Geometry: final body of the model. Coordinates: model frame, mm. A direction names the side the tool comes from. Round coordinates to 2 decimals unless told otherwise and drop trailing zeros. Loops run counter-clockwise (first coordinate to the right, second up) from the corner with the lowest first, then second, coordinate; pieces in that order, holes last. Notation, with made-up numbers: M 12,52.5 L 60,52.5 A20 cw 60,83.5 Z; hole C -9.5,54.25 d5. An arc over 180 degrees is marked long. Return JSON: item names as keys, results as strings.
from build123d import *

# Parameters (mm, degrees)
CROQUIS1_W                 = 45
CROQUIS1_H                 = 45
SALIENTE_EXTRUIR1_DEPTH    = 300
CROQUIS4_W                 = 18
CROQUIS4_H                 = 34
CORTAR_EXTRUIR2_DEPTH      = 46
CROQUIS8_W                 = 35
CROQUIS8_H                 = 35
CORTAR_EXTRUIR3_DEPTH      = 301
CROQUIS9_W                 = 35
CROQUIS9_H                 = 21.174410022
CORTAR_EXTRUIR4_DEPTH      = 10
CROQUIS10_R                = 1
CORTAR_EXTRUIR5_DEPTH      = 10
CROQUIS11_W                = 45
CROQUIS11_H                = 26.387879272
CORTAR_EXTRUIR6_DEPTH      = 46
CROQUIS13_W                = 45
CROQUIS13_H                = 50
CORTAR_EXTRUIR7_DEPTH      = 23.5
CORTAR_EXTRUIR7_DEPTH_BACK = 23.5
CROQUIS14_W                = 55
CROQUIS14_H                = 55
SALIENTE_EXTRUIR2_DEPTH    = 5
CROQUIS16_R                = 1
CORTAR_EXTRUIR8_DEPTH      = 1
CORTAR_EXTRUIR8_DEPTH_BACK = 229.612120728
CROQUIS17_R                = 2.5
CROQUIS17_R_2              = 2.03
CORTAR_EXTRUIR9_DEPTH      = 6
CORTAR_EXTRUIR9_DEPTH_BACK = 51


with BuildPart() as part:
    # Croquis1 → Saliente-Extruir1 (new body)
    with BuildSketch(Plane(origin=(0, 0, 0), x_dir=(1, 0, 0), z_dir=(0, 1, 0))):
        Rectangle(CROQUIS1_W, CROQUIS1_H)
    extrude(amount=SALIENTE_EXTRUIR1_DEPTH)

    # Croquis4 → Cortar-Extruir2 (cut, through all)
    with BuildSketch(Plane.ZY.offset(22.5)):
        with Locations((13.5, 17)):
            Rectangle(CROQUIS4_W, CROQUIS4_H)
    extrude(amount=-CORTAR_EXTRUIR2_DEPTH, mode=Mode.SUBTRACT)

    # Croquis8 → Cortar-Extruir3 (cut, through all)
    with BuildSketch(Plane(origin=(0, 300, 0), x_dir=(1, 0, 0), z_dir=(0, 1, 0))):
        Rectangle(CROQUIS8_W, CROQUIS8_H)
    extrude(amount=-CORTAR_EXTRUIR3_DEPTH, mode=Mode.SUBTRACT)

    # Croquis9 → Cortar-Extruir4 (cut)
    with BuildSketch(Plane(origin=(0, 0, -22.5), x_dir=(-1, 0, 0), z_dir=(0, 0, -1))):
        with Locations((0, 260)):
            Rectangle(CROQUIS9_W, CROQUIS9_H)
    extrude(amount=-CORTAR_EXTRUIR4_DEPTH, mode=Mode.SUBTRACT)

    # Croquis10 → Cortar-Extruir5 (cut)
    with BuildSketch(Plane.XY.offset(22.5)):
        with Locations((0, 260)):
            Circle(CROQUIS10_R)
    extrude(amount=-CORTAR_EXTRUIR5_DEPTH, mode=Mode.SUBTRACT)

    # Croquis11 → Cortar-Extruir6 (cut, through all)
    with BuildSketch(Plane.XY.offset(22.5)):
        with Locations((0, 286.806060364)):
            Rectangle(CROQUIS11_W, CROQUIS11_H)
    extrude(amount=-CORTAR_EXTRUIR6_DEPTH, mode=Mode.SUBTRACT)

    # Croquis13 → Cortar-Extruir7 (cut, two sides)
    with BuildSketch(Plane(origin=(0, 0, 0), x_dir=(0, 0, -1), z_dir=(1, 0, 0))) as cortar_extruir7_sk:
        with Locations((0, 25)):
            Rectangle(CROQUIS13_W, CROQUIS13_H)
    extrude(amount=CORTAR_EXTRUIR7_DEPTH, mode=Mode.SUBTRACT)
    extrude(cortar_extruir7_sk.sketch, amount=-CORTAR_EXTRUIR7_DEPTH_BACK, mode=Mode.SUBTRACT)

    # Croquis14 → Saliente-Extruir2 (add)
    with BuildSketch(Plane.XZ.offset(-50)):
        Rectangle(CROQUIS14_W, CROQUIS14_H)
    extrude(amount=SALIENTE_EXTRUIR2_DEPTH)

    # Croquis16 → Cortar-Extruir8 (cut, two sides)
    with BuildSketch(Plane.XZ.offset(-45)) as cortar_extruir8_sk:
        with Locations((25, 25)):
            Circle(CROQUIS16_R)
        with Locations((-25, 25)):
            Circle(CROQUIS16_R)
        with Locations((-25, -25)):
            Circle(CROQUIS16_R)
        with Locations((25, -25)):
            Circle(CROQUIS16_R)
    extrude(amount=CORTAR_EXTRUIR8_DEPTH, mode=Mode.SUBTRACT)
    extrude(cortar_extruir8_sk.sketch, amount=-CORTAR_EXTRUIR8_DEPTH_BACK, mode=Mode.SUBTRACT)

    # Croquis17 → Cortar-Extruir9 (cut, two sides)
    with BuildSketch(Plane.XY.offset(22.5)) as cortar_extruir9_sk:
        with Locations((-10, 262.50260741)):
            Circle(CROQUIS17_R)
        with Locations((-10, 206.50260741)):
            Circle(CROQUIS17_R)
        with Locations((10, 262.50260741)):
            Circle(CROQUIS17_R)
        with Locations((10, 206.50260741)):
            Circle(CROQUIS17_R)
        with Locations((10, 254.10260741)):
            Circle(CROQUIS17_R_2)
        with Locations((10, 214.90260741)):
            Circle(CROQUIS17_R_2)
    extrude(amount=CORTAR_EXTRUIR9_DEPTH, mode=Mode.SUBTRACT)
    extrude(cortar_extruir9_sk.sketch, amount=-CORTAR_EXTRUIR9_DEPTH_BACK, mode=Mode.SUBTRACT)


solid = part.part
Q1. Pin query (flat end, axial travel): pin 1 (6 mm diameter, centred on x = -10, y = 262.5, fed in from +Z); pin 2 (10 mm diameter, centred on y = 186.5, z = -21.5, fed in from -X); pin 3 (10 mm diameter, centred on y = 156.5, z = 6.5, fed in from +X). Return the tip coordinate at first contact, or that it passes through.
Determined:
{"pin 1": "stops at z = 22.5", "pin 2": "stops at x = -22.5", "pin 3": "stops at x = 22.5"}
Q2. Section query D-D (z = -20.5). Output: boundary loops of the cut face in (x, y), plus the area to 3 significant figures.
Determined:
{"outline": "M -27.5,45 L 27.5,45 L 27.5,50 L 22.5,50 L 22.5,273.61 L -22.5,273.61 L -22.5,50 L -27.5,50 Z; hole M -17.5,249.41 L 17.5,249.41 L 17.5,270.59 L -17.5,270.59 Z; hole C -10,206.5 d5; hole C 10,206.5 d5; hole C 10,214.9 d4.06", "area": "9,540 mm^2"}
Q3. Pull-direction query (Y, two-part tool) for faces 1 (the flat face through (0, 249.413, -20)), 2 (the flat face through (0, 160, 22.5)), 3 (the flat face through (20, 273.612, 0)); classes: pulls with the +Y half, pulls with the -Y half, needs draft (parallel to the pull), parting line crosses it, or undercut.
Determined:
{"face 1": "undercut", "face 2": "needs draft", "face 3": "pulls with the +Y half"}
Q4. Section query A-A (y = 196). Output: boundary loops of the cut face in (x, z).
Determined:
{"outline": "M -22.5,-22.5 L 22.5,-22.5 L 22.5,22.5 L -22.5,22.5 Z; hole M -17.5,-17.5 L 17.5,-17.5 L 17.5,17.5 L -17.5,17.5 Z"}
Q5. Section query B-B (z = 2.5). Output: boundary loops of the cut face in (x, y).
Determined:
{"outline": "M -27.5,45 L 27.5,45 L 27.5,50 L 22.5,50 L 22.5,273.61 L 17.5,273.61 L 17.5,50 L -17.5,50 L -17.5,273.61 L -22.5,273.61 L -22.5,50 L -27.5,50 Z"}
Q6. Reachability of faces 4 (the flat face through (0, 151, -17.5)), 5 (the flat face through (-22.5, 160, 0)), 6 (the flat face through (0, 160, -22.5)), 7 (the flat face through (0, 270.587, -20)) from +Z, -Z, +X, -X, +Y, -Y: full face, straight path, thin tool, end or side. Return the list, or none.
Determined:
{"face 4": "+Y", "face 5": "+Z, -Z, -X, +Y", "face 6": "-Z, +X, -X, +Y", "face 7": "-Z"}
Q7. Section query C-C (x = 10). State how many separate pieces and enclosed holes the cut face has, plus the area to 3 significant figures.
Determined:
{"separate pieces": "8", "enclosed holes": "0", "area": "2,270 mm^2"}
Q8. Material intervals for L1, parallel to Y at x = 10, z = -19; L2, parallel to Y at x = -10, z = 20; L3, parallel to Z at x = -25, y = 46.45, sorted ascending.
Determined:
{"L1": "y = 45 to 204, 209 to 212.87, 216.93 to 249.41, 270.59 to 273.61", "L2": "y = 45 to 204, 209 to 260, 265 to 273.61", "L3": "z = -27.5 to -26, -24 to 24, 26 to 27.5"}
